Can you work these out from the model? Positions are in its coordinate system, mm. Coordinates: 2 decimals unless noted, no trailing zeros. Order: outer loops, then holes, each group sorted by start corner. A loop starts at its lowest first (then second) coordinate and runs counter-clockwise, first axis right, second up. Notation, with made-up numbers: M 32.25,-0.75 L 47.25,-0.75 A29 ccw 47.25,28.25 Z; hole C 53,48.5 d11. An arc over 180 degrees is marked long. Answer as a JSON object with one key per item and string values.
from build123d import *

# Parameters (mm, degrees)
SKETCH1_W               = 76
SKETCH1_H               = 63
SKETCH1_R               = 6.05
SKETCH1_R_2             = 1.6
BOSS_EXTRUDE1_DEPTH     = 3.175
CHAMFER1_SIZE           = 4
F_1_4_20_TAPPED_HOLE1_D = 5.1054


with BuildPart() as part:
    # Sketch1 → Boss-Extrude1 (new body)
    with BuildSketch(Plane.XY):
        with Locations((6, -14.99999999)):
            Rectangle(SKETCH1_W, SKETCH1_H)
        with Locations((-7, 0)):
            Circle(SKETCH1_R, mode=Mode.SUBTRACT)
        with Locations((-13.423393759, 7.75)):
            Circle(SKETCH1_R_2, mode=Mode.SUBTRACT)
        with Locations((-13.423393759, -7.75)):
            Circle(SKETCH1_R_2, mode=Mode.SUBTRACT)
        with Locations((0, -15.5)):
            Circle(SKETCH1_R_2, mode=Mode.SUBTRACT)
        with Locations((13.423393759, -7.75)):
            Circle(SKETCH1_R_2, mode=Mode.SUBTRACT)
        with Locations((13.423393759, 7.75)):
            Circle(SKETCH1_R_2, mode=Mode.SUBTRACT)
    extrude(amount=BOSS_EXTRUDE1_DEPTH)

    # Chamfer1
    chamfer1_edges = [part.edges().sort_by_distance(p)[0] for p in [
        (-32, 16.50000001, 1.5875),
        (44, 16.50000001, 1.5875),
        (44, -46.49999999, 1.5875),
        (-32, -46.49999999, 1.5875),
    ]]
    chamfer(chamfer1_edges, length=CHAMFER1_SIZE)

    # 1/4-20 Tapped Hole1 (through all)
    with Locations(Plane.XY.offset(3.175)):
        with Locations((-24, 9.50000001), (36, 9.50000001), (36, -40.49999999), (-24, -40.49999999)):
            Hole(F_1_4_20_TAPPED_HOLE1_D / 2)


solid = part.part
Item 1: If we mould it in two halves opening along Y, with no side actions, what happens to faces 1 (the cylindrical face through (-0.208, -13.914, 1.565)), 2 (the cylindrical face through (-11.945, 7.137, 1.565)), 3 (the flat face through (42, -44.5, 1.6)), 4 (the flat face through (44, -15, 2))? For each: pulls with the +Y half, pulls with the -Y half, needs draft (parallel to the pull), parting line crosses it, or undercut.
Answers follow:
{"face 1": "undercut", "face 2": "undercut", "face 3": "pulls with the -Y half", "face 4": "needs draft"}
Item 2: I want a section at B-B, the plane y = 0. Write out the boundary of the cut face in (x, z) (3 decimals), plus the area to 3 significant figures.
Answers follow:
{"outline": "M -32,0 L -13.05,0 L -13.05,3.175 L -32,3.175 Z; M -0.95,0 L 44,0 L 44,3.175 L -0.95,3.175 Z", "area": "203 mm^2"}
Item 3: I want a section at D-D, the plane z = 1.6. Give the number of separate pieces and of enclosed holes in the cut face, plus the area to 3 significant figures.
Answers follow:
{"separate pieces": "1", "enclosed holes": "10", "area": "4,520 mm^2"}
Item 4: I'm going to push a flat-ended pin straight in: pin 1 (9.5 mm diameter, centred on x = -7, y = 0, fed in from -Z). Where does the tip first touch, or does it pass through?
Answers follow:
{"pin 1": "passes through"}
Item 5: I want a section at A-A, the plane x = 36. Write out the boundary of the cut face in (y, z) (3 decimals), plus the area to 3 significant figures.
Answers follow:
{"outline": "M -46.5,0 L -43.053,0 L -43.053,3.175 L -46.5,3.175 Z; M -37.947,0 L 6.947,0 L 6.947,3.175 L -37.947,3.175 Z; M 12.053,0 L 16.5,0 L 16.5,3.175 L 12.053,3.175 Z", "area": "168 mm^2"}
Item 6: I want a section at C-C, the plane y = -40.5. Write out the boundary of the cut face in (x, z) (3 decimals), plus the area to 3 significant figures.
Answers follow:
{"outline": "M -32,0 L -26.553,0 L -26.553,3.175 L -32,3.175 Z; M -21.447,0 L 33.447,0 L 33.447,3.175 L -21.447,3.175 Z; M 38.553,0 L 44,0 L 44,3.175 L 38.553,3.175 Z", "area": "209 mm^2"}
Item 7: Please list where these lines run through material, in increasing order: line 1 (Y direction, x = -24, z = 2.25); line 2 (X direction, y = -7, z = 3.05); line 3 (X direction, y = 8.5, z = 2.15).
Answers follow:
{"line 1": "y = -46.5 to -43.05, -37.95 to 6.95, 12.05 to 16.5", "line 2": "x = -32 to -14.84, -12.01 to 12.01, 14.84 to 44", "line 3": "x = -32 to -26.35, -21.65 to -14.84, -12.01 to 12.01, 14.84 to 33.65, 38.35 to 44"}
